```python
from build123d import *

# Parameters (mm, degrees)
MODEL_R             = 0.5
MODEL_R_2           = 0.75
BOSS_EXTRUDE1_DEPTH = 2


with BuildPart() as part:
    # Model → Boss-Extrude1 (new body)
    with BuildSketch(Plane.XY):
        with BuildLine():
            Line((1967.109841287, 1238.384705077), (1983.109841287, 1238.384705077))
            ThreePointArc((1983.109841287, 1238.384705077), (1984.524054849, 1238.970491514), (1985.109841287, 1240.384705077))
            Line((1985.109841287, 1240.384705077), (1985.109841287, 1243.384705077))
            Line((1985.109841287, 1243.384705077), (1978.859841287, 1243.384705077))
            Line((1978.859841287, 1243.384705077), (1978.859841287, 1245.384705077))
            Line((1978.859841287, 1245.384705077), (1985.109841287, 1245.384705077))
            Line((1985.109841287, 1245.384705077), (1985.109841287, 1272.584705077))
            Line((1985.109841287, 1272.584705077), (1978.859841287, 1272.584705077))
            Line((1978.859841287, 1272.584705077), (1978.859841287, 1274.584705077))
            Line((1978.859841287, 1274.584705077), (1985.109841287, 1274.584705077))
            Line((1985.109841287, 1274.584705077), (1985.109841287, 1276.584705077))
            ThreePointArc((1985.109841287, 1276.584705077), (1983.645375192, 1280.120238983), (1980.109841287, 1281.584705077))
            Line((1980.109841287, 1281.584705077), (1970.109841287, 1281.584705077))
            ThreePointArc((1970.109841287, 1281.584705077), (1966.574307381, 1280.120238983), (1965.109841287, 1276.584705077))
            Line((1965.109841287, 1276.584705077), (1965.109841287, 1274.584705077))
            Line((1965.109841287, 1274.584705077), (1971.359841287, 1274.584705077))
            Line((1971.359841287, 1274.584705077), (1971.359841287, 1272.584705077))
            Line((1971.359841287, 1272.584705077), (1965.109841287, 1272.584705077))
            Line((1965.109841287, 1272.584705077), (1965.109841287, 1245.384705077))
            Line((1965.109841287, 1245.384705077), (1971.359841287, 1245.384705077))
            Line((1971.359841287, 1245.384705077), (1971.359841287, 1243.384705077))
            Line((1971.359841287, 1243.384705077), (1965.109841287, 1243.384705077))
            Line((1965.109841287, 1243.384705077), (1965.109841287, 1240.384705077))
            ThreePointArc((1965.109841287, 1240.384705077), (1965.695627724, 1238.970491514), (1967.109841287, 1238.384705077))
        make_face()
        with Locations((1968.109841287, 1278.584705077)):
            Circle(MODEL_R, mode=Mode.SUBTRACT)
        with Locations((1982.109841287, 1278.584705077)):
            Circle(MODEL_R, mode=Mode.SUBTRACT)
        with Locations((1979.109841287, 1247.884705077)):
            Circle(MODEL_R_2, mode=Mode.SUBTRACT)
        with Locations((1971.109841287, 1247.884705077)):
            Circle(MODEL_R_2, mode=Mode.SUBTRACT)
        with Locations((1979.109841287, 1270.084705077)):
            Circle(MODEL_R_2, mode=Mode.SUBTRACT)
        with Locations((1971.109841287, 1270.084705077)):
            Circle(MODEL_R_2, mode=Mode.SUBTRACT)
        with Locations((1982.359841287, 1240.884705077)):
            Circle(MODEL_R_2, mode=Mode.SUBTRACT)
        with Locations((1967.859841287, 1240.884705077)):
            Circle(MODEL_R_2, mode=Mode.SUBTRACT)
    extrude(amount=BOSS_EXTRUDE1_DEPTH)


solid = part.part
```
The model under review builds one solid part; all positions refer to its coordinate system, in mm. A direction names the side the tool comes from. Coordinates: 2 decimals unless noted, no trailing zeros. Write each loop counter-clockwise with the first axis right and the second up, starting at its lowest first coordinate (ties: lowest second). Pieces come first, ordered by that corner, then holes. Notation, with made-up numbers: (-39.5, 39.25) -> (-26.5, 39.25) arc R25 ccw to (-26.5, 55.25) -> close; hole circle Ø2 at (-11, 62). An arc over 180 degrees is marked (long way). One line per item, written item: value. Start each with the question number.
Q1. The part is to be moulded in two halves that separate along Y. For faces 4 (the face through (1978.86, 1244, 1)), 5 (the face through (1966.613, 1280.159, 0.986)), 6 (the face through (1985.11, 1259, 1)), say which applies: +Y half, -Y half, draft (parallel to the pull), parting line (faces both ways), or undercut.
Q2. Clearance check with flat-ended pins moving along their axes: P1, Ø0.6, axis at x = 1982.5, z = 0.5, coming from the +Y side; P2, Ø1, axis at y = 1274, z = 1.5, coming from the -X side. State where each tip first meets the part, or that it passes through.
Q3. Add section B-B, the plane x = 1980.5. Give the boundary of the cut face in (y, z), then the cut area to 3 significant figures.
Q4. For faces 1 (the face through (1975, 1238.385, 1)), 2 (the face through (1971.36, 1274, 1)), 3 (the face through (1982, 1243.385, 1)), list the 3-axis set-ups (+Z, -Z, +X, -X, +Y, -Y) from which the entire face can be reached by the end or side of a thin tool; tool diameter is ignored.
Q5. Add section A-A, the plane z = 1.25. Count the separate pieces of the cut face and the enclosed holes in it, then the cut area to 3 significant figures.
Q6. To check wall thickness, follow probe 1 along Y at (x, z) = (1980.5, 1.25); probe 2 along Y at (x, z) = (1971.75, 1); probe 3 along X at (y, z) = (1247.5, 1). State the ranges of each line that lie inside material, in increasing order.
Response:
1. face 4: undercut
1. face 5: +Y half
1. face 6: draft
2. P1: y = 1281.13
2. P2: x = 1971.36
3. outline: (1238.38, 0) -> (1243.38, 0) -> (1243.38, 2) -> (1238.38, 2) -> close; (1245.38, 0) -> (1272.58, 0) -> (1272.58, 2) -> (1245.38, 2) -> close; (1274.58, 0) -> (1281.57, 0) -> (1281.57, 2) -> (1274.58, 2) -> close
3. area: 78.4 mm²
4. face 1: +Z, -Z, +X, -X, -Y
4. face 2: +Z, -Z, -X
4. face 3: +Z, -Z, +X
5. separate pieces: 1
5. enclosed holes: 8
5. area: 789 mm²
6. probe 1: 1238.38 to 1243.38, 1245.38 to 1272.58, 1274.58 to 1281.57
6. probe 2: 1238.38 to 1247.49, 1248.28 to 1269.69, 1270.48 to 1281.58
6. probe 3: 1965.11 to 1970.47, 1971.75 to 1978.47, 1979.75 to 1985.11
